For this review, take the finished solid that the model builds, in its own axes (mm). A direction names the side the tool comes from. Coordinates: 2 decimals unless noted, no trailing zeros. Write each loop counter-clockwise with the first axis right and the second up, starting at its lowest first coordinate (ties: lowest second). Pieces come first, ordered by that corner, then holes. Notation, with made-up numbers: (-24.75, -12.5) -> (23.25, -12.5) arc R8 ccw to (23.25, -4.5) -> close; hole circle Ø3 at (57.5, 17). An arc over 180 degrees is marked (long way). Put each result on its own line as item: value. Start each with the question number.
Item 1: Consider section C-C on x = 0. Give the boundary of the cut face in (y, z).
Item 2: Consider section D-D on z = 64. Give the boundary of the cut face in (x, y).
Item 3: Consider section B-B on x = 22.5. Give the boundary of the cut face in (y, z), and give its area (3 significant figures).
Item 4: To check wall thickness, follow L1, parallel to Z at x = 22, y = -22; L2, parallel to X at y = 3.5, z = 36; L3, parallel to X at y = -11.5, z = 69. State the ranges of each line that lie inside material, in increasing order.
Item 5: For faces 1 (the flat face through (-21.3, 12.53, 9.93)), 2 (the flat face through (-21.501, -12.183, 9.93)), 3 (the conical face through (-2.928, -13.184, 55.56)), 4 (the flat face through (0, -24.712, 10)), 5 (the flat face through (21.501, 12.183, 9.93)), list the 3-axis set-ups (+Z, -Z, +X, -X, +Y, -Y) from which the entire face can be reached by the end or side of a thin tool; tool diameter is ignored.
Item 6: Insertion check: P1, Ø1.5, axis at x = 3, z = 24.5, coming from the -Y side; P2, Ø3, axis at x = 5, z = 10.5, coming from the -Y side; P3, Ø5, axis at y = 9, z = 37.5, coming from the +X side. Each pin has a flat end and moves straight along its axis. Give the tip position at first contact, or say it passes through.
Item 7: Consider section A-A on z = 6.5. Give the boundary of the cut face in (x, y), and give its area (3 significant figures).
Item 8: The part is to be moulded in two halves that separate along Z. For faces 6 (the flat face through (12, 0, 15)), 7 (the flat face through (0, 24.712, 10)), 8 (the flat face through (-1, 0, 0)), say which applies: +Z half, -Z half, draft (parallel to the pull), parting line (faces both ways), or undercut.
```python
from build123d import *

# Parameters (mm, degrees)
F0_W     = 87.9223719239
F0_H     = 69.4261789322
F1_DEPTH = 5
F3_DEPTH = 10
F4_R     = 9.9566569638
F5_DEPTH = 80
F5_TAPER = -5


with BuildPart() as f1:
    # F0 (on Top) → F1 (new body)
    with BuildSketch(Plane.XY):
        Rectangle(F0_W, F0_H)
    extrude(amount=F1_DEPTH)

    # F2 (on face) → F3 (join)
    with BuildSketch(Plane.XY.offset(5)):
        Polygon((14.2674572932, 24.7119609267), (-14.2674572932, 24.7119609267), (-28.5349145864, 0), (-14.2674572932, -24.7119609267), (14.2674572932, -24.7119609267), (28.5349145864, 0), align=None)
    extrude(amount=F3_DEPTH)

    # F4 (on face) → F5 (join)
    with BuildSketch(Plane.XY.offset(15)):
        Circle(F4_R)
    extrude(amount=F5_DEPTH, taper=F5_TAPER)


solid = f1.part
```
Return value:
1. outline: (-34.71, 0) -> (34.71, 0) -> (34.71, 5) -> (24.71, 5) -> (24.71, 15) -> (9.96, 15) -> (16.96, 95) -> (-16.96, 95) -> (-9.96, 15) -> (-24.71, 15) -> (-24.71, 5) -> (-34.71, 5) -> close
2. outline: circle Ø28.49 at (0, 0)
3. outline: (-34.71, 0) -> (34.71, 0) -> (34.71, 5) -> (10.45, 5) -> (10.45, 15) -> (-10.45, 15) -> (-10.45, 5) -> (-34.71, 5) -> close
3. area: 556 mm^2
4. L1: 0 to 5
4. L2: -11.26 to 11.26
4. L3: -9.13 to 9.13
5. face 1: +Z, -X, +Y
5. face 2: +Z, -X, -Y
5. face 3: none
5. face 4: +Z, +X, -X, -Y
5. face 5: +Z, +X, +Y
6. P1: y = -10.56
6. P2: y = -24.71
6. P3: x = 10.02
7. outline: (-28.53, 0) -> (-14.27, -24.71) -> (14.27, -24.71) -> (28.53, 0) -> (14.27, 24.71) -> (-14.27, 24.71) -> close
7. area: 2,120 mm^2
8. face 6: undercut
8. face 7: draft
8. face 8: -Z half
